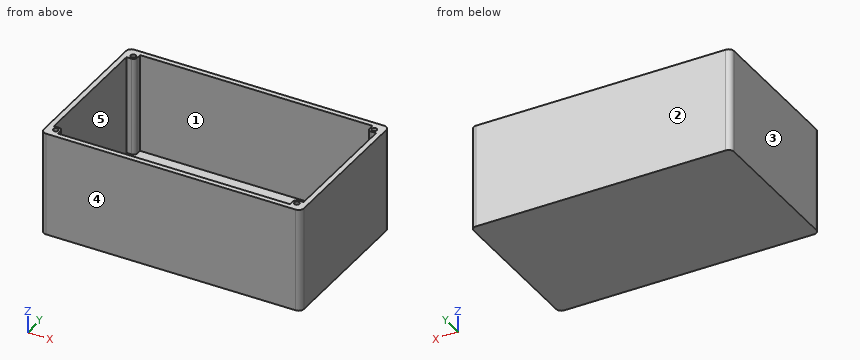
from build123d import *

# Parameters (mm, degrees)
F0_W     = 144
F0_H     = 84
F1_DEPTH = 3
F0_W_2   = 150
F0_H_2   = 90
F2_DEPTH = 60
F3_R     = 3
F4_W     = 5
F4_H     = 5
F5_DEPTH = 57
F6_R     = 1.5
F7_DEPTH = 30
F8_R     = 2


with BuildPart() as f1:
    # F0 (on Top) → F1 (new body)
    with BuildSketch(Plane.XY):
        with Locations((4.453997, -2.561509)):
            Rectangle(F0_W, F0_H)
    extrude(amount=F1_DEPTH)

    # F0 (on Top) → F2 (join)
    with BuildSketch(Plane.XY):
        with Locations((4.453997, -2.561509)):
            Rectangle(F0_W_2, F0_H_2)
        with Locations((4.453997, -2.561509)):
            Rectangle(F0_W, F0_H, mode=Mode.SUBTRACT)
    extrude(amount=F2_DEPTH)

    # F3
    f3_edges = [f1.edges().sort_by_distance(p)[0] for p in [
        (-70.546003, 42.438491, 30),
        (-70.546003, -47.561509, 30),
        (79.453997, -47.561509, 30),
        (79.453997, 42.438491, 30),
    ]]
    fillet(f3_edges, radius=F3_R)

    # F4 (on face) → F5 (join)
    with BuildSketch(Plane.XY.offset(3)):
        with Locations((-65.046003, 36.938491)):
            Rectangle(F4_W, F4_H)
        with Locations((-65.046003, -42.061509)):
            Rectangle(F4_W, F4_H)
        with Locations((73.953997, 36.938491)):
            Rectangle(F4_W, F4_H)
        with Locations((73.953997, -42.061509)):
            Rectangle(F4_W, F4_H)
    extrude(amount=F5_DEPTH)

    # F6 (on face) → F7 (cut)
    with BuildSketch(Plane.XY.offset(60)):
        with Locations((-65.046003, 36.938491)):
            Circle(F6_R)
        with Locations((-65.046003, -42.061509)):
            Circle(F6_R)
        with Locations((73.953997, -42.061509)):
            Circle(F6_R)
        with Locations((73.953997, 36.938491)):
            Circle(F6_R)
    extrude(amount=-F7_DEPTH, mode=Mode.SUBTRACT)

    # F8
    f8_edges = [f1.edges().sort_by_distance(p)[0] for p in [
        (-62.546003, 34.438491, 31.5),
        (71.453997, 34.438491, 31.5),
        (71.453997, -39.561509, 31.5),
        (-62.546003, -39.561509, 31.5),
    ]]
    fillet(f8_edges, radius=F8_R)


solid = f1.part
Check sheet for the modelled part. Datum: model origin and axes. Units: mm. Face numbers are marked on the shaded views. A direction names the side the tool comes from. Give positions to 0.01 mm unless a question says otherwise; leave off trailing zeros. Write each loop counter-clockwise with the first axis right and the second up, starting at its lowest first coordinate (ties: lowest second). Pieces come first, ordered by that corner, then holes. Notation, with made-up numbers: (-38, 77) -> (-15, 77) arc R20 cw to (-15, 110) -> close; hole circle Ø1 at (-9, -37.5). An arc over 180 degrees is marked (long way). One line per item, written item: value. Start each with the question number.
Item 1: Draft check along Y on the marked faces 3, 4 and 5. Enter one of: +Y half, -Y half, draft (parallel to the pull), parting line (faces both ways), or undercut.
Item 2: Section check A-A on z = 9. Record the cut outline in (x, y), then the cut area to 3 significant figures.
Item 3: Section check D-D on z = 34.5. Record the cut outline in (x, y).
Item 4: Gauge pin test, flat ends, axial feed: pin 1 (2.5 mm diameter, centred on x = -65.05, y = 36.94, fed in from +Z); pin 2 (5 mm diameter, centred on x = -49, y = 20, fed in from +Z). Record the tip position at first contact, or that the pin passes through.
Item 5: Material ranges on probe 1 along X at (y, z) = (-42, 55.5); probe 2 along Y at (x, z) = (65.5, 36); probe 3 along X at (y, z) = (34, 27.5), recorded low to high. Write a range as from..to.
Item 6: Section check B-B on y = 8. Record the cut outline in (x, z), then the cut area to 3 significant figures.
Item 7: Section check C-C on x = -30. Record the cut outline in (y, z), then the cut area to 3 significant figures.
Item 8: Tool access check on the marked faces 1 and 2. Record the directions out of +Z, -Z, +X, -X, +Y, -Y that give a thin tool (end or side, any length) a straight path to the whole face; none if there is none.
Results list:
1. face 3: draft
1. face 4: -Y half
1. face 5: undercut
2. outline: (-70.55, -44.56) arc R3 ccw to (-67.55, -47.56) -> (76.45, -47.56) arc R3 ccw to (79.45, -44.56) -> (79.45, 39.44) arc R3 ccw to (76.45, 42.44) -> (-67.55, 42.44) arc R3 ccw to (-70.55, 39.44) -> close; hole (-67.55, -39.56) -> (-64.55, -39.56) arc R2 cw to (-62.55, -41.56) -> (-62.55, -44.56) -> (71.45, -44.56) -> (71.45, -41.56) arc R2 cw to (73.45, -39.56) -> (76.45, -39.56) -> (76.45, 34.44) -> (73.45, 34.44) arc R2 cw to (71.45, 36.44) -> (71.45, 39.44) -> (-62.55, 39.44) -> (-62.55, 36.44) arc R2 cw to (-64.55, 34.44) -> (-67.55, 34.44) -> close
2. area: 1,490 mm²
3. outline: (-70.55, -44.56) arc R3 ccw to (-67.55, -47.56) -> (76.45, -47.56) arc R3 ccw to (79.45, -44.56) -> (79.45, 39.44) arc R3 ccw to (76.45, 42.44) -> (-67.55, 42.44) arc R3 ccw to (-70.55, 39.44) -> close; hole (-67.55, -39.56) -> (-64.55, -39.56) arc R2 cw to (-62.55, -41.56) -> (-62.55, -44.56) -> (71.45, -44.56) -> (71.45, -41.56) arc R2 cw to (73.45, -39.56) -> (76.45, -39.56) -> (76.45, 34.44) -> (73.45, 34.44) arc R2 cw to (71.45, 36.44) -> (71.45, 39.44) -> (-62.55, 39.44) -> (-62.55, 36.44) arc R2 cw to (-64.55, 34.44) -> (-67.55, 34.44) -> close; hole circle Ø3 at (-65.05, -42.06); hole circle Ø3 at (-65.05, 36.94); hole circle Ø3 at (73.95, -42.06); hole circle Ø3 at (73.95, 36.94)
4. pin 1: z = 30
4. pin 2: z = 3
5. probe 1: -70.55..-66.54, -63.55..-62.55, 71.45..72.46, 75.45..79.45
5. probe 2: -47.56..-44.56, 39.44..42.44
5. probe 3: -70.55..-67.55, 76.45..79.45
6. outline: (-70.55, 0) -> (79.45, 0) -> (79.45, 60) -> (76.45, 60) -> (76.45, 3) -> (-67.55, 3) -> (-67.55, 60) -> (-70.55, 60) -> close
6. area: 792 mm²
7. outline: (-47.56, 0) -> (42.44, 0) -> (42.44, 60) -> (39.44, 60) -> (39.44, 3) -> (-44.56, 3) -> (-44.56, 60) -> (-47.56, 60) -> close
7. area: 612 mm²
8. face 1: +Z
8. face 2: +Z, -Z, +X, -X, +Y
